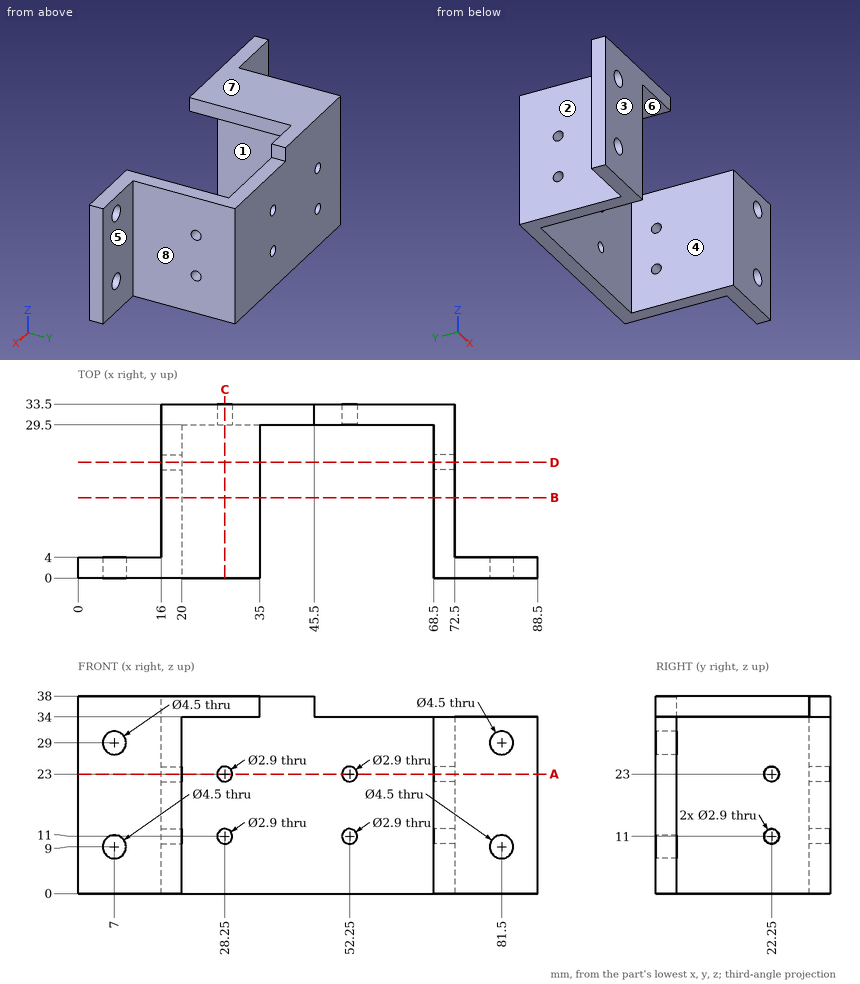
Geometry: see drawing. Coordinates: mm, zero at the bounding-box minimum. A direction names the side the tool comes from. Round coordinates to 2 decimals unless told otherwise and drop trailing zeros. Loops run counter-clockwise (first coordinate to the right, second up) from the corner with the lowest first, then second, coordinate; pieces in that order, holes last. Notation, with made-up numbers: M -16,4 L 39,4 A24 cw 39,18 Z; hole C 86,-27 d5. An arc over 180 degrees is marked long. Use a Markdown table: item, result. Add a question column.
1. Line query: line 1 (X direction, y = 2, z = 9); line 2 (Z direction, x = 28.25, y = 32.55); line 3 (X direction, y = 30.6, z = 11). Output: solid intervals per line, ascending.
2. Mould query, pull axis X, two halves, no side actions, for the marked faces 6, 7 and 8. Classes: pulls with the +X half, pulls with the -X half, needs draft (parallel to the pull), parting line crosses it, or undercut.
3. Section query B-B on y = 15.5. Return the cut outline in (x, z), then the cut area to 3 significant figures.
4. Section query D-D on y = 22.25. Return the cut outline in (x, z), then the cut area to 3 significant figures.
5. Section query C-C on x = 28.25. Return the cut outline in (y, z).
6. Reachability of the marked faces 1, 2, 3, 4 and 5 from +Z, -Z, +X, -X, +Y, -Y: full face, straight path, thin tool, end or side. Return the list, or none.
7. Section query A-A on z = 23. Return the cut outline in (x, y), then the cut area to 3 significant figures.
8. Contact query for flat-ended pins moving along their axis: P1, Ø10, axis at y = 25.5, z = 14, coming from the -X side; P2, Ø3.5, axis at x = 52.25, z = 23, coming from the -Y side; P3, Ø6, axis at x = 7, z = 29, coming from the +Y side; P4, Ø2, axis at x = 72.5, y = 20, coming from the -Z side. Output: stop coordinate, or through.
Reported:
| question | item | result |
|---|---|---|
| 1 | line 1 | x = 0 to 4.75, 9.25 to 20, 68.5 to 79.25, 83.75 to 88.5 |
| 1 | line 2 | z = 0 to 9.55, 12.45 to 21.55, 24.45 to 38 |
| 1 | line 3 | x = 16 to 26.8, 29.7 to 50.8, 53.7 to 72.5 |
| 2 | face 6 | undercut |
| 2 | face 7 | needs draft |
| 2 | face 8 | pulls with the +X half |
| 3 | outline | M 16,0 L 20,0 L 20,34 L 35,34 L 35,38 L 16,38 Z; M 68.5,0 L 72.5,0 L 72.5,34 L 68.5,34 Z |
| 3 | area | 348 mm² |
| 4 | outline | M 16,0 L 20,0 L 20,9.55 L 16,9.55 Z; M 16,12.45 L 20,12.45 L 20,21.55 L 16,21.55 Z; M 16,24.45 L 20,24.45 L 20,34 L 35,34 L 35,38 L 16,38 Z; M 68.5,0 L 72.5,0 L 72.5,9.55 L 68.5,9.55 Z; M 68.5,12.45 L 72.5,12.45 L 72.5,21.55 L 68.5,21.55 Z; M 68.5,24.45 L 72.5,24.45 L 72.5,34 L 68.5,34 Z |
| 4 | area | 302 mm² |
| 5 | outline | M 0,34 L 29.5,34 L 29.5,24.45 L 33.5,24.45 L 33.5,38 L 0,38 Z; M 29.5,0 L 33.5,0 L 33.5,9.55 L 29.5,9.55 Z; M 29.5,12.45 L 33.5,12.45 L 33.5,21.55 L 29.5,21.55 Z |
| 6 | face 1 | -Z, -Y |
| 6 | face 2 | +Z, -Z, -X, +Y |
| 6 | face 3 | +Z, -Z, +X, -X, -Y |
| 6 | face 4 | +Z, -Z, -Y |
| 6 | face 5 | +Z, -Z, +X, +Y |
| 7 | outline | M 0,0 L 20,0 L 20,20.8 L 16,20.8 L 16,4 L 0,4 Z; M 16,23.7 L 20,23.7 L 20,29.5 L 26.8,29.5 L 26.8,33.5 L 16,33.5 Z; M 29.7,29.5 L 50.8,29.5 L 50.8,33.5 L 29.7,33.5 Z; M 53.7,29.5 L 68.5,29.5 L 68.5,23.7 L 72.5,23.7 L 72.5,33.5 L 53.7,33.5 Z; M 68.5,0 L 88.5,0 L 88.5,4 L 72.5,4 L 72.5,20.8 L 68.5,20.8 Z |
| 7 | area | 544 mm² |
| 8 | P1 | stops at x = 16 |
| 8 | P2 | stops at y = 29.5 |
| 8 | P3 | stops at y = 4 |
| 8 | P4 | stops at z = 0 |
